Design review of the part built by this model. Coordinates are the model's own, in mm. A direction names the side the tool comes from. Round coordinates to 2 decimals unless told otherwise and drop trailing zeros. Order: outer loops, then holes, each group sorted by start corner. A loop starts at its lowest first (then second) coordinate and runs counter-clockwise, first axis right, second up. Notation, with made-up numbers: (-15, 61.5) - (-10, 61.5) arc R15 cw to (-10, 83.5) - close; hole circle Ø8 at (-36, 67). An arc over 180 degrees is marked (long way). Write item = value, one per line.
Autodesk Inventor part; units mm, degrees
ref_plane "YZ Plane" through (0, 0, 0) normal (1, 0, 0) x (0, 1, 0)
ref_plane "XZ Plane" through (0, 0, 0) normal (0, 1, 0) x (-1, 0, 0)
ref_plane "XY Plane" through (0, 0, 0) normal (0, 0, 1) x (1, 0, 0)
sketch "Sketch1" plane through (0, 0, 0) normal (0, 1, 0) x (-1, 0, 0)
  line L0 (600, 0) -> (-600, 0)
  line L1 (-600, 0) -> (-600, 600)
  line L2 (-600, 600) -> (600, 600)
  line L3 (600, 600) -> (600, 0)
  point P0 (0, 0)
  point P1 (0, 0)
  dimension "d0" = 1200
  dimension "d1" = 600
extrude "Extrusion1" add sketch "Sketch1" along normal blind 850
sketch "Sketch2" plane through (0, 850, 0) normal (0, 1, 0) x (1, 0, 0)
  line L0 (-425, -500) -> (425, -500)
  line L1 (425, -500) -> (425, -100)
  line L2 (425, -100) -> (-425, -100)
  line L3 (-425, -100) -> (-425, -500)
  line L4 (-425, -500) -> (425, -100) construction
  line L5 (425, -500) -> (-425, -100) construction
  line L6 (-600, 0) -> (-600, -600)
  line L7 (-600, -600) -> (600, -600)
  point P0 (0, 0)
  point P1 (0, -300)
  point P2 (-600, -300)
  point P3 (-600, -300)
  point P4 (0, -600)
  dimension "d4" = 850
  dimension "d5" = 400
extrude "Extrusion2" cut sketch "Sketch2" against normal blind 180
fillet "Fillet1" radius 20 8 edges at (-425, 760, 100) (-425, 670, 300) (0, 670, 100) (-425, 760, 500) (0, 670, 500) (425, 670, 300) (425, 760, 500) (425, 760, 100)
sketch "Sketch3" plane through (-600, 0, 600) normal (0, 0, 1) x (1, 0, 0)
  line L0 (0, 0) -> (1200, 0)
  line L1 (1200, 0) -> (1200, 850)
  line L2 (0, 0) -> (1200, 0)
  line L3 (1200, 0) -> (1200, 120)
  line L4 (1200, 120) -> (0, 120)
  line L5 (0, 120) -> (0, 0)
  point P0 (600, 0)
  dimension "d9" = 120
extrude "Extrusion3" cut sketch "Sketch3" against normal blind 20
sketch "Sketch4" plane through (0, 0, 0) normal (1, 0, 0) x (0, 1, 0)
  line L0 (850, 120) -> (850, 100)
  line L1 (850, 120) -> (850, 480)
  line L2 (850, 500) -> (850, 480)
  line L3 (850, 480) -> (850, 500)
  line L4 (850, 480) -> (850, 120)
  line L5 (850, 100) -> (850, 120)
  line L6 (850, 600) -> (850, 0)
  line L7 (850, 0) -> (850, 600)
  line L8 (850, 50) -> (1020, 50)
  arc A0 (1020, 50) -> (1050, 80) centre (1020, 80) ccw
  line L9 (1050, 80) -> (1050, 220)
  arc A1 (1050, 220) -> (1020, 250) centre (1020, 220) ccw
  line L10 (1020, 250) -> (990, 250)
  point P0 (0, 0)
  dimension "d12" = 60
  dimension "d13" = 200
  dimension "d14" = 50
  dimension "d15" = 200
  dimension "d16" = 30
sketch "Sketch5" plane through (0, 850, 0) normal (0, 1, 0) x (1, 0, 0)
  circle A0 centre (0, -50) radius 15
  point P0 (0, 0)
  dimension "d17" = 30
sweep "Sweep1" add profiles "Sketch5" path "Sketch4" path curves L8 A0 L9 A1 L10
properties part number "Mobile lavandino 1200"
Item 1: Take a section at A-A, the plane z = 156. State the section outline as (x, y) points.
Data:
outline = (-600, 0) - (600, 0) - (600, 850) - (425, 850) - (425, 690) arc R20 cw to (405, 670) - (-405, 670) arc R20 cw to (-425, 690) - (-425, 850) - (-600, 850) - close; circle Ø30 at (0, 1050)
Item 2: Take a section at D-D, the plane x = -343. State the section outline as (y, z) points.
Data:
outline = (0, 0) - (850, 0) - (850, 100) - (690, 100) arc R20 cw to (670, 120) - (670, 480) arc R20 cw to (690, 500) - (850, 500) - (850, 600) - (120, 600) - (120, 580) - (0, 580) - close
Item 3: For faces 1 (the face through (-1.953, 936.19, 35.128)), 2 (the face through (-8, 61, 580)), 3 (the face through (0, 990, 250)), 4 (the face through (425, 771, 303)), list the 3-axis set-ups (+Z, -Z, +X, -X, +Y, -Y) from which the entire face can be reached by the end or side of a thin tool; tool diameter is ignored.
Data:
face_1 = none
face_2 = +Z, +X, -X, -Y
face_3 = +Z, +X, -X
face_4 = +Y
Item 4: The part is to be moulded in two halves that separate along X. For faces 5 (the face through (8, 0, 294)), 6 (the face through (6, 771, 100)), 7 (the face through (-600, 419, 304)), say which applies: +X half, -X half, draft (parallel to the pull), parting line (faces both ways), or undercut.
Data:
face_5 = draft
face_6 = undercut
face_7 = -X half
Item 5: For line 1 along X through (y, z) = (827, 279); line 2 along Z through (x, y) = (23, 788); line 3 along Z through (x, y) = (-26, 113), list the stretches that pass through material, from the lowest coordinate up. Write a range as [from, to].
Data:
line_1 = [-600, -425], [425, 600]
line_2 = [0, 100], [500, 600]
line_3 = [0, 580]
Item 6: Take a section at C-C, the plane z = 410.5. State the section outline as (x, y) points, and give its area (3 significant figures).
Data:
outline = (-600, 0) - (600, 0) - (600, 850) - (425, 850) - (425, 690) arc R20 cw to (405, 670) - (-405, 670) arc R20 cw to (-425, 690) - (-425, 850) - (-600, 850) - close
area = 867,000 mm2
Item 7: Take a section at B-B, the plane x = 0. State the section outline as (y, z) points, and give its area (3 significant figures).
Data:
outline = (0, 0) - (850, 0) - (850, 35) - (1020, 35) arc R45 ccw to (1065, 80) - (1065, 220) arc R45 ccw to (1020, 265) - (990, 265) - (990, 235) - (1020, 235) arc R15 cw to (1035, 220) - (1035, 80) arc R15 cw to (1020, 65) - (850, 65) - (850, 100) - (690, 100) arc R20 cw to (670, 120) - (670, 480) arc R20 cw to (690, 500) - (850, 500) - (850, 600) - (120, 600) - (120, 580) - (0, 580) - close
area = 449,000 mm2
Item 8: Insertion check: P1, Ø6, axis at x = 61, z = 589, coming from the -Y side; P2, Ø10, axis at x = -374.5, z = 343.5, coming from the +Y side. Each pin has a flat end and moves straight along its axis. Give the tip position at first contact, or say it passes through.
Data:
P1 = 120
P2 = 670
